Could you check a few things on this model? Use its own coordinates, in mm. A direction names the side the tool comes from. Coordinates: 2 decimals unless noted, no trailing zeros. Write each loop counter-clockwise with the first axis right and the second up, starting at its lowest first coordinate (ties: lowest second). Pieces come first, ordered by that corner, then holes. Notation, with made-up numbers: (76.25, 86) - (105.25, 86) arc R23 cw to (105.25, 114) - close; hole circle Ø7 at (-2, 47.5). An arc over 180 degrees is marked (long way). Answer as a JSON object with one key per item and string values. Group by question number.
1) Will these pins go through, and if not, where does the flat tip stop? pin 1 Ø6 at (y, z) = (9, -36.5) entering from +X; pin 2 Ø2 at (y, z) = (16.5, -38) entering from +X; pin 3 Ø6 at (x, z) = (-8, -31.5) entering from -Y; pin 4 Ø13.5 at (x, y) = (0, 0) entering from +Z.
2) On a 3-axis mill with a long thin cutter (end or side, diameter ignored), from which of +Z, -Z, +X, -X, +Y, -Y can I reach the whole of each face in a straight line? I mean faces 4 (the cylindrical face through (16.128, -25.296, -32.023)), 5 (the flat face through (-2, -9, -7.3)), 6 (the cylindrical face through (1.172, -8.923, -32.049)), 7 (the flat face through (-9, 8, 0)), 8 (the flat face through (2, -9, -57.5)). Say none if no direction works.
3) If we section it at A-A (z = -30): Write out the boundary of the cut face in (x, y), plus the area to 3 significant figures.
4) Please list where these lines run through material, in increasing order: line 1 along Z through (x, y) = (-28, 21); line 2 along Y through (x, z) = (0, -37); line 3 along Y through (x, z) = (0, -1).
5) We'd pull the mould along X, two halves only. Please class faces 1 (the cylindrical face through (-8.238, 37.096, -2.472)), 2 (the flat face through (9, 8, -64.8)), 3 (the cylindrical face through (-5.97, -9.36, -3.6)): released by +X, released by -X, zero draft, split by the parting line, or undercut.
```python
from build123d import *

# Parameters (mm, degrees)
CHAMFER1_SIZE = 0.5


with BuildPart() as part:
    # Sketch1 → Revolve1 (revolve)
    with BuildSketch(Plane(origin=(0, 0, 0), x_dir=(1, 0, 0), z_dir=(0, 1, 0)), mode=Mode.PRIVATE) as revolve1_sk:
        Polygon((0, 0), (0, 64.8), (-38, 64.8), (-38, 59.8), (-30, 59.8), (-30, 5), (-38, 5), (-38, 0), align=None)
    revolve(revolve1_sk.sketch.rotate(Axis((0, 0, 0), (0, 0, -1)), 180), axis=Axis((0, 0, 0), (0, 0, -1)))

    # Sketch7 → Cut-Revolve1 (revolve, cut)
    with BuildSketch(Plane(origin=(0, 0, 0), x_dir=(1, 0, 0), z_dir=(0, 1, 0))):
        Polygon((0, 64.8), (-11.1, 64.8), (-11.1, 57.5), (-9, 57.5), (-9, 7.3), (-11.1, 7.3), (-11.1, 0), (0, 0), align=None)
    revolve(axis=Axis((0, 0, -64.8), (0, 0, 1)), mode=Mode.SUBTRACT)

    # Chamfer1
    chamfer1_edges = [part.edges().sort_by_distance(p)[0] for p in [
        (-38, 0, 0),
        (-38, 0, -5),
        (-30, 0, -5),
        (-30, 0, -59.8),
        (-38, 0, -59.8),
        (-38, 0, -64.8),
    ]]
    chamfer(chamfer1_edges, length=CHAMFER1_SIZE)


solid = part.part
```
Here are the results:
{
 "1": {"pin 1": "stops at x = 29.39", "pin 2": "stops at x = 25.69", "pin 3": "stops at y = -29.58", "pin 4": "passes through"},
 "2": {"face 4": "none", "face 5": "+Z", "face 6": "+Z, -Z", "face 7": "+Z, +X, -X, +Y, -Y", "face 8": "-Z"},
 "3": {"outline": "circle Ø60 at (0, 0); hole circle Ø18 at (0, 0)", "area": "2,570 mm²"},
 "4": {"line 1": "z = -64.8 to -59.8, -5 to 0", "line 2": "y = -30 to -9, 9 to 30", "line 3": "y = -38 to -11.1, 11.1 to 38"},
 "5": {"face 1": "split by the parting line", "face 2": "zero draft", "face 3": "undercut"}
}
